Source: CAD feature listing. Evaluate the final solid. Frame: model axes, mm. A direction names the side the tool comes from. Give positions to 0.01 mm unless a question says otherwise; leave off trailing zeros. Loops run counter-clockwise (first coordinate to the right, second up) from the corner with the lowest first, then second, coordinate; pieces in that order, holes last. Notation, with made-up numbers: M 76,-9.5 L 108,-9.5 A28 ccw 108,27.5 Z; hole C 56,-18.5 d11. An arc over 180 degrees is marked long. Answer in a Markdown table with one row per item.
```python
from build123d import *

# Parameters (mm, degrees)
PAD002_DEPTH = 5.2
SKETCH006_R  = 1.05
PAD003_DEPTH = 1.6
PAD003_TAPER = 30
SKETCH007_W  = 30
SKETCH007_H  = 6
PAD004_DEPTH = 4.8


with BuildPart() as part:
    # Sketch005 → Pad002 (new body)
    with BuildSketch(Plane.XZ):
        Polygon((-20.2, -1.5), (-18.352479, 1.7), (-2.581495, 1.7), (-3.851666, 3.9), (-0.651666, 3.9), (0.618505, 1.7), (5.5, 1.7), (5.5, -1.5), (8, -1.5), (8, 4.5), (-22, 4.5), (-22, -1.5), align=None)
    extrude(amount=PAD002_DEPTH)

    # Sketch006 → Pad003 (join)
    with BuildSketch(Plane.XZ.offset(5.2)):
        Circle(SKETCH006_R)
    extrude(amount=-PAD003_DEPTH, taper=PAD003_TAPER)

    # Sketch007 → Pad004 (join)
    with BuildSketch(Plane.XZ.offset(5.2)):
        with Locations((-7, 1.5)):
            Rectangle(SKETCH007_W, SKETCH007_H)
    extrude(amount=PAD004_DEPTH)


solid = part.part
```
1) Pin query (flat end, axial travel): pin 1 Ø1.6 at (x, y) = (-9.5, -2.5) entering from -Z; pin 2 Ø3.5 at (x, y) = (-3, -3.5) entering from -Z. Return the tip coordinate at first contact, or that it passes through.
Reply:
| item | result |
|---|---|
| pin 1 | stops at z = 1.7 |
| pin 2 | stops at z = -1.5 |
2) Section B-B, the plane y = -0.5. Return loops of the section in (x, z).
Reply:
| item | result |
|---|---|
| outline | M -22,-1.5 L -20.2,-1.5 L -18.35,1.7 L -2.58,1.7 L -3.85,3.9 L -0.65,3.9 L 0.62,1.7 L 5.5,1.7 L 5.5,-1.5 L 8,-1.5 L 8,4.5 L -22,4.5 Z |
3) Material intervals for L1, parallel to X at y = -4, z = 0; L2, parallel to X at y = -4.25, z = 3.2; L3, parallel to X at y = -1.25, z = 1.65, sorted ascending.
Reply:
| item | result |
|---|---|
| L1 | x = -22 to -19.33, -0.36 to 0.36, 5.5 to 8 |
| L2 | x = -22 to -3.45, -0.25 to 8 |
| L3 | x = -22 to -18.38, 5.5 to 8 |
4) Section A-A, the plane x = -8. Return loops of the section in (y, z).
Reply:
| item | result |
|---|---|
| outline | M -10,-1.5 L -5.2,-1.5 L -5.2,1.7 L 0,1.7 L 0,4.5 L -10,4.5 Z |
5) Set-up query: faces 1 (the flat face through (5.5, -3, 0)), 2 (the flat face through (-7, -10, 2)), 3 (the flat face through (-3.208, -2.564, 2.785)). Return all of +Z, -Z, +X, -X, +Y, -Y with unobstructed straight access to the full face (end or side cutting, diameter ignored); none if empty.
Reply:
| item | result |
|---|---|
| face 1 | -Z, +Y |
| face 2 | +Z, -Z, +X, -X, -Y |
| face 3 | +Y |
6) Pull-direction query (Z, two-part tool) for faces 4 (the flat face through (-7, -5, 4.5)), 5 (the flat face through (-7, 0, 2)), 6 (the flat face through (-11, -3, 1.7)), 7 (the flat face through (-2, -3, 3.9)); classes: released by +Z, released by -Z, zero draft, split by the parting line, or undercut.
Reply:
| item | result |
|---|---|
| face 4 | released by +Z |
| face 5 | zero draft |
| face 6 | released by -Z |
| face 7 | undercut |
7) Section C-C, the plane z = 3.25. Return loops of the section in (x, y).
Reply:
| item | result |
|---|---|
| outline | M -22,-10 L 8,-10 L 8,0 L -0.28,0 L -0.28,-5.2 L -3.48,-5.2 L -3.48,0 L -22,0 Z |
